Autodesk Inventor part; units mm, degrees
ref_plane "YZ Plane" through (0, 0, 0) normal (1, 0, 0) x (0, 1, 0)
ref_plane "XZ Plane" through (0, 0, 0) normal (0, 1, 0) x (-1, 0, 0)
ref_plane "XY Plane" through (0, 0, 0) normal (0, 0, 1) x (1, 0, 0)
sketch "Sketch1" plane through (0, 0, 0) normal (0, 0, 1) x (1, 0, 0)
  line L0 (-50, -60) -> (50, -60)
  line L1 (50, -60) -> (50, 60)
  line L2 (50, 60) -> (-50, 60)
  line L3 (-50, 60) -> (-50, -60)
  line L4 (-50, -60) -> (50, 60) construction
  line L5 (50, -60) -> (-50, 60) construction
  point P0 (0, 0)
  dimension "d0" = 100
  dimension "d1" = 120
extrude "Plate1" add sketch "Sketch1" along normal blind 6.35
sketch "Sketch2" plane through (-43.65, -60, 0) normal (-1, 0, 0) x (0, -1, 0)
  line L0 (-120, 0) -> (0, 0)
  line L1 (0, 0) -> (0, 110)
  line L2 (0, 110) -> (-120, 110)
  line L3 (-120, 110) -> (-120, 0)
edge flange "Flange1" height 110 angle 90 thickness 6.35 bend radius 6.35 thickness toward (-1, 0, 0) relief tear relief width 6.35 relief depth 3.175 corner gap 6.35 corner form 0 edges at (-50, 0, 6.35) (50, 0, 6.35) wall of the first edge with corners at (-43.65, 60, 0) (-43.65, -60, 0) (-43.65, -60, 110) (-43.65, 60, 110)
bend "Bend1"
corner "Corner1"
sketch "Sketch3" plane through (50, -60, 110) normal (1, 0, 0) x (0, 0, -1)
  circle A0 centre (30, 60) radius 21.082 construction
  circle A1 centre (30, 60) radius 21.5
  point P0 (110, 60)
  dimension "d13" = 42.164
  dimension "d14" = 43
  dimension "d15" = 80
extrude "Cut1" cut sketch "Sketch3" against normal through all
sketch "Sketch4" plane through (0, 0, 6.35) normal (0, 0, 1) x (1, 0, 0)
  circle A0 centre (0, 0) radius 15.5
  dimension "d18" = 31
extrude "Cut2" cut sketch "Sketch4" against normal blind 6.35
sketch "Sketch5" plane through (50, -60, 110) normal (1, 0, 0) x (0, 0, -1)
  circle A0 centre (30, 60) radius 21.5
  line L0 (97.3, 0) -> (97.3, 120)
  line L1 (0, 120) -> (97.3, 120)
  line L2 (0, 0) -> (0, 120)
  line L3 (97.3, 0) -> (0, 0)
  line L4 (0, 120) -> (97.3, 120) construction
  line L5 (97.3, 0) -> (0, 0) construction
  line L6 (17.542, 105.5) -> (17.542, 14.5) construction
  line L7 (0, 0) -> (0, 120) construction
  point P0 (110, 60)
  point P1 (0, 60)
  point P2 (17.542, 60)
  dimension "d38" = 17.542
  dimension "d39" = 45.5
hole "Hole1" at (50, -45.5, 92.458) at (50, 45.5, 92.458) direction (-1, 0, 0) diameter 6.6 end through all
sketch "Sketch6" plane through (50, -60, 110) normal (1, 0, 0) x (0, 0, -1)
  circle A0 centre (17.542, 14.5) radius 3.3
  circle A1 centre (17.542, 105.5) radius 3.3
  circle A2 centre (30, 60) radius 21.5
  line L0 (97.3, 0) -> (97.3, 120)
  line L1 (0, 120) -> (97.3, 120)
  line L2 (0, 0) -> (0, 120)
  line L3 (97.3, 0) -> (0, 0)
  line L4 (83.542, 25) -> (83.542, 95) construction
  point P0 (110, 60)
  point P1 (83.542, 60)
  dimension "d29" = 70
  dimension "d30" = 83.542
hole "Hole2" at (50, -35, 26.458) at (50, 35, 26.458) direction (-1, 0, 0) diameter 4.5 end through all
equation "\"d16\" = Thickness"
equation "\"d19\" = Thickness"
equation "\"d27\" = Thickness"
equation "\"d36\" = Thickness"
equation "\"d2\" = Thickness"
equation "\"d3\" = BendReliefWidth"
equation "\"d4\" = BendReliefDepth"
equation "\"d5\" = MinimumRemnant"
equation "\"d6\" = TransitionRadius"
equation "\"d9\" = BendRadius"
equation "\"d10\" = CornerReliefSize"
equation "\"d11\" = GapSize"
equation "\"d12\" = JacobiRadiusSize"
equation "\"BendRadius\" = Thickness"
equation "\"BendReliefWidth\" = Thickness"
equation "\"BendReliefDepth\" = 0.5 * Thickness"
equation "\"CornerReliefSize\" = 4 * Thickness"
equation "\"MinimumRemnant\" = 2 * Thickness"
equation "\"TransitionRadius\" = BendRadius"
equation "\"JacobiRadiusSize\" = BendRadius"
equation "\"GapSize\" = Thickness"
properties part number "Ground_Tracker_Bearing" material "UHMW, White"
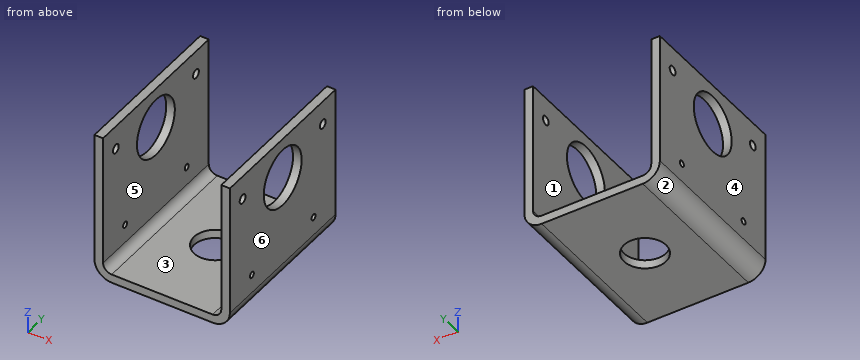
CAD build for the part. Positions are in the model's coordinates, mm. Face numbers are marked on the shaded views. A direction names the side the tool comes from. Give positions to 0.01 mm unless a question says otherwise; leave off trailing zeros. Order: outer loops, then holes, each group sorted by start corner. A loop starts at its lowest first (then second) coordinate and runs counter-clockwise, first axis right, second up. Notation, with made-up numbers: (45.5, -11) -> (88.5, -11) arc R8 ccw to (88.5, 3) -> close; hole circle Ø6 at (-39, 5). An arc over 180 degrees is marked (long way). Return JSON: item names as keys, results as strings.
Q1. Saw through at C-C (z = 31). Write the cut outline in (x, y).
Working result:
{"outline": "(-50, -60) -> (-43.65, -60) -> (-43.65, 60) -> (-50, 60) -> close; (43.65, -60) -> (50, -60) -> (50, 60) -> (43.65, 60) -> close"}
Q2. Which spindle directions (+Z, -Z, +X, -X, +Y, -Y) get a long thin tool onto all of the face, cutting with end or side? Do the marked faces 1 and 2. Say none if no direction does.
Working result:
{"face 1": "+Z, +Y, -Y", "face 2": "-Z, -X, +Y, -Y"}
Q3. Saw through at D-D (y = 28). Write the cut outline in (x, z), then the cut area to 3 significant figures.
Working result:
{"outline": "(-50, 12.7) arc R12.7 ccw to (-37.3, 0) -> (37.3, 0) arc R12.7 ccw to (50, 12.7) -> (50, 110) -> (43.65, 110) -> (43.65, 12.7) arc R6.35 cw to (37.3, 6.35) -> (-37.3, 6.35) arc R6.35 cw to (-43.65, 12.7) -> (-43.65, 110) -> (-50, 110) -> close", "area": "1,900 mm²"}
Q4. Saw through at B-B (x = 0). Write the cut outline in (y, z).
Working result:
{"outline": "(-60, 0) -> (-15.5, 0) -> (-15.5, 6.35) -> (-60, 6.35) -> close; (15.5, 0) -> (60, 0) -> (60, 6.35) -> (15.5, 6.35) -> close"}
Q5. Drill centre lines: line 1 (X direction, y = -49, z = 32); line 2 (Y direction, x = 45, z = 80); line 3 (Z direction, x = -4, y = 32). Where is each one in solid material? Low to high.
Working result:
{"line 1": "-50 to -43.65, 43.65 to 50", "line 2": "-60 to -21.5, 21.5 to 60", "line 3": "0 to 6.35"}
Q6. Flat gauge pin, fed straight in: pin 1 (22.5 mm diameter, centred on x = 7, y = 20, fed in from +Z). Where does the tip first touch, or does it go through?
Working result:
{"pin 1": "z = 6.35"}
Q7. Mould opens along X. For the marked faces 3, 4, 5 and 6 say: pulls with the +X half, pulls with the -X half, needs draft (parallel to the pull), parting line crosses it, or undercut.
Working result:
{"face 3": "undercut", "face 4": "pulls with the -X half", "face 5": "undercut", "face 6": "pulls with the +X half"}
Q8. Saw through at A-A (y = 45.5). Write the cut outline in (x, z).
Working result:
{"outline": "(-50, 12.7) arc R12.7 ccw to (-37.3, 0) -> (37.3, 0) arc R12.7 ccw to (50, 12.7) -> (50, 89.16) -> (43.65, 89.16) -> (43.65, 12.7) arc R6.35 cw to (37.3, 6.35) -> (-37.3, 6.35) arc R6.35 cw to (-43.65, 12.7) -> (-43.65, 89.16) -> (-50, 89.16) -> close; (-50, 95.76) -> (-43.65, 95.76) -> (-43.65, 110) -> (-50, 110) -> close; (43.65, 95.76) -> (50, 95.76) -> (50, 110) -> (43.65, 110) -> close"}
